Geometry check sheet. Reference: the model listing, model coordinates, mm. A direction names the side the tool comes from. Round coordinates to 2 decimals unless told otherwise and drop trailing zeros. Order: outer loops, then holes, each group sorted by start corner. A loop starts at its lowest first (then second) coordinate and runs counter-clockwise, first axis right, second up. Notation, with made-up numbers: (-15, 59.25) - (29, 59.25) arc R19 cw to (29, 87.25) - close; hole circle Ø1 at (87.5, -23). An arc over 180 degrees is marked (long way). Answer as CSV lines item,"result". Start each with the question number.
```python
from build123d import *

# Parameters (mm, degrees)
CYLINDER050_R          = 14.5
CYLINDER050_DEPTH      = 22
CYLINDER050_ROLL_ANGLE = 90
CYLINDER047_R          = 1.8
CYLINDER047_DEPTH      = 10
CYLINDER048_R          = 1.2
CYLINDER048_DEPTH      = 10
CYLINDER048_ROLL_ANGLE = 90
CYLINDER049_R          = 1.2
CYLINDER049_DEPTH      = 10
CYLINDER049_ROLL_ANGLE = 90
CYLINDER046_R          = 1.8
CYLINDER046_DEPTH      = 10
BOX006_W               = 52
BOX006_H               = 13
BOX006_DEPTH           = 40
BOX012_W               = 80
BOX012_H               = 20
BOX012_DEPTH           = 4
CYLINDER035_R          = 4.2
CYLINDER035_DEPTH      = 200
BOX007_W               = 25
BOX007_H               = 27
BOX007_DEPTH           = 20
CHAMFER007_SIZE        = 5
CHAMFER008_SIZE        = 5
CHAMFER009_SIZE        = 2
CHAMFER010_SIZE        = 5
CHAMFER011_SIZE        = 5
CHAMFER012_SIZE        = 5
CHAMFER013_SIZE        = 5
CHAMFER014_SIZE        = 5


with BuildPart() as cilindro047:
    # Cylinder050 → Cylinder050 (new body)
    with BuildSketch(Plane.XY):
        Circle(CYLINDER050_R)
    extrude(amount=CYLINDER050_DEPTH)


with BuildPart() as cilindro047_1:
    # Cylinder050 roll: moved
    add(cilindro047.part.rotate(Axis((0, 0, 0), (1, 0, 0)), CYLINDER050_ROLL_ANGLE))


with BuildPart() as cilindro047_2:
    # Cylinder050 placement: moved
    add(cilindro047_1.part.moved(Location((88, -7, -1))))


with BuildPart() as cilindro044:
    # Cylinder047 → Cylinder047 (new body)
    with BuildSketch(Plane(origin=(52, -15, -35), x_dir=(1, 0, 0), z_dir=(0, 0, 1))):
        Circle(CYLINDER047_R)
    extrude(amount=CYLINDER047_DEPTH)


with BuildPart() as cilindro045:
    # Cylinder048 → Cylinder048 (new body)
    with BuildSketch(Plane.XY):
        Circle(CYLINDER048_R)
    extrude(amount=CYLINDER048_DEPTH)


with BuildPart() as cilindro045_1:
    # Cylinder048 roll: moved
    add(cilindro045.part.rotate(Axis((0, 0, 0), (1, 0, 0)), CYLINDER048_ROLL_ANGLE))


with BuildPart() as cilindro045_2:
    # Cylinder048 placement: moved
    add(cilindro045_1.part.moved(Location((70.5, -17, -1))))


with BuildPart() as cilindro046:
    # Cylinder049 → Cylinder049 (new body)
    with BuildSketch(Plane.XY):
        Circle(CYLINDER049_R)
    extrude(amount=CYLINDER049_DEPTH)


with BuildPart() as cilindro046_1:
    # Cylinder049 roll: moved
    add(cilindro046.part.rotate(Axis((0, 0, 0), (1, 0, 0)), CYLINDER049_ROLL_ANGLE))


with BuildPart() as cilindro046_2:
    # Cylinder049 placement: moved
    add(cilindro046_1.part.moved(Location((105.5, -17, -1))))


with BuildPart() as fusion010:
    # Cylinder046 → Cylinder046 (new body)
    with BuildSketch(Plane(origin=(119, -18, -35), x_dir=(1, 0, 0), z_dir=(0, 0, 1))):
        Circle(CYLINDER046_R)
    extrude(amount=CYLINDER046_DEPTH)

    # Fusion010: union Cilindro044, Cilindro045, Cilindro046
    add(cilindro044.part)
    add(cilindro045_2.part)
    add(cilindro046_2.part)


with BuildPart() as cubo006:
    # Box006 → Box006 (new body)
    with BuildSketch(Plane(origin=(62, -26, -34), x_dir=(1, 0, 0), z_dir=(0, 0, 1))):
        with Locations((26, 6.5)):
            Rectangle(BOX006_W, BOX006_H)
    extrude(amount=BOX006_DEPTH)


with BuildPart() as cubo012:
    # Box012 → Box012 (new body)
    with BuildSketch(Plane(origin=(44, -29, -34), x_dir=(1, 0, 0), z_dir=(0, 0, 1))):
        with Locations((40, 10)):
            Rectangle(BOX012_W, BOX012_H)
    extrude(amount=BOX012_DEPTH)


with BuildPart() as cilindro032:
    # Cylinder035 → Cylinder035 (new body)
    with BuildSketch(Plane(origin=(57, -40, -29), x_dir=(1, 0, 0), z_dir=(0, 0, 1))):
        Circle(CYLINDER035_R)
    extrude(amount=CYLINDER035_DEPTH)


with BuildPart() as base_motor:
    # Box007 → Box007 (new body)
    with BuildSketch(Plane(origin=(44, -49, -34), x_dir=(1, 0, 0), z_dir=(0, 0, 1))):
        with Locations((12.5, 13.5)):
            Rectangle(BOX007_W, BOX007_H)
    extrude(amount=BOX007_DEPTH)

    # Cut028: cut Cilindro032
    add(cilindro032.part, mode=Mode.SUBTRACT)

    # Fusion011: union Cubo006, Cubo012
    add(cubo006.part)
    add(cubo012.part)

    # Cut035: cut Fusion010
    add(fusion010.part, mode=Mode.SUBTRACT)

    # Cut036: cut Cilindro047
    add(cilindro047_2.part, mode=Mode.SUBTRACT)

    # Chamfer007
    chamfer007_edges = [base_motor.edges().sort_by_distance(p)[0] for p in [
        (69, -37.5, -14),
    ]]
    chamfer(chamfer007_edges, length=CHAMFER007_SIZE)

    # Chamfer008
    chamfer008_edges = [base_motor.edges().sort_by_distance(p)[0] for p in [
        (62, -17.5, -30),
    ]]
    chamfer(chamfer008_edges, length=CHAMFER008_SIZE)

    # Chamfer009
    chamfer009_edges = [base_motor.edges().sort_by_distance(p)[0] for p in [
        (114, -19.5, -30),
    ]]
    chamfer(chamfer009_edges, length=CHAMFER009_SIZE)

    # Chamfer010
    chamfer010_edges = [base_motor.edges().sort_by_distance(p)[0] for p in [
        (44, -22, -22),
    ]]
    chamfer(chamfer010_edges, length=CHAMFER010_SIZE)

    # Chamfer011
    chamfer011_edges = [base_motor.edges().sort_by_distance(p)[0] for p in [
        (44, -49, -24),
    ]]
    chamfer(chamfer011_edges, length=CHAMFER011_SIZE)

    # Chamfer012
    chamfer012_edges = [base_motor.edges().sort_by_distance(p)[0] for p in [
        (62, -19.5, 6),
    ]]
    chamfer(chamfer012_edges, length=CHAMFER012_SIZE)

    # Chamfer013
    chamfer013_edges = [base_motor.edges().sort_by_distance(p)[0] for p in [
        (114, -19.5, 6),
    ]]
    chamfer(chamfer013_edges, length=CHAMFER013_SIZE)

    # Chamfer014
    chamfer014_edges = [base_motor.edges().sort_by_distance(p)[0] for p in [
        (69, -49, -26.5),
    ]]
    chamfer(chamfer014_edges, length=CHAMFER014_SIZE)


solid = base_motor.part
```
1. Thickness scan on probe 1 along X at (y, z) = (-18.75, -1); probe 2 along Y at (x, z) = (119, -33.2); probe 3 along Y at (x, z) = (57, -20). Record the ranges inside material, lowest first.
2. Section check A-A on y = -18. Record the boundary of the cut face in (x, z), plus the area to 3 significant figures.
3. Draft check along Y on faces 1 (the face through (117.2, -17.92, -32.03)), 2 (the face through (54, -35, -14)), 3 (the face through (46, -46, -24)). Enter one of: released by +Y, released by -Y, zero draft, split by the parting line, or undercut.
4. Section check B-B on z = -26. Record the boundary of the cut face in (x, y).
5. Section check C-C on x = 88. Record the boundary of the cut face in (y, z), plus the area to 4 significant figures.
6. Go/stop test with flat-tipped pins: pin 1 Ø1.9 at (x, z) = (70.5, -1) entering from -Y; pin 2 Ø14.5 at (y, z) = (-21.5, -13) entering from +X; pin 3 Ø1 at (y, z) = (-25, -23.5) entering from -X; pin 4 Ø6 at (x, y) = (119, -18) entering from -Z. Record where each tip stops, or that it passes through.
7. Section check D-D on x = 52. Record the boundary of the cut face in (y, z).
8. Access from +Z, -Z, +X, -X, +Y, -Y to the whole of each face (thin tool, end or side, straight path). Record for faces 4 (the face through (105, -17, -1)), 5 (the face through (86, -13, -16)), 6 (the face through (46, -25, -22)), 7 (the face through (67, -38, -17)), 8 (the face through (114, -20, -14)).
Numbers:
1,probe 1,"x = 62 to 69.3, 71.7 to 73.5, 102.5 to 104.3, 106.7 to 114"
1,probe 2,"y = -29 to -19.8, -16.2 to -9"
1,probe 3,"y = -49 to -44.2, -35.8 to -22"
2,outline,"(44, -34) - (117.2, -34) - (117.2, -30) - (116, -30) - (114, -28) - (114, 1) - (109, 6) - (100.7, 6) arc R14.5 cw (long way) to (75.3, 6) - (67, 6) - (62, 1) - (62, -25) - (57, -30) - (44, -30) - close; (120.8, -34) - (124, -34) - (124, -30) - (120.8, -30) - close; hole circle Ø2.4 at (70.5, -1); hole circle Ø2.4 at (105.5, -1)"
2,area,"1,630 mm2"
3,face 1,"undercut"
3,face 2,"zero draft"
3,face 3,"released by -Y"
4,outline,"(44, -44) - (49, -49) - (64, -49) - (69, -44) - (69, -26) - (114, -26) - (114, -13) - (61, -13) - (61, -22) - (49, -22) - (44, -27) - close; hole circle Ø8.4 at (57, -40)"
5,outline,"(-29, -34) - (-9, -34) - (-9, -30) - (-13, -30) - (-13, -15.5) - (-26, -15.5) - (-26, -30) - (-29, -30) - close"
5,area,"268.5 mm2"
6,pin 1,"stops at y = -17"
6,pin 2,"stops at x = 114"
6,pin 3,"stops at x = 45.5"
6,pin 4,"stops at z = -34"
7,outline,"(-49, -34) - (-16.8, -34) - (-16.8, -30) - (-22, -30) - (-22, -14) - (-49, -14) - close; (-13.2, -34) - (-9, -34) - (-9, -30) - (-13.2, -30) - close"
8,face 4,"-Y"
8,face 5,"+Z, +X, -X, +Y"
8,face 6,"+Z, -X, +Y"
8,face 7,"+Z, +X, -Y"
8,face 8,"+Z, +X, +Y, -Y"
